Can you work these out from the drawing? Everything is in mm from the part's minimum corner. A direction names the side the tool comes from. Coordinates: 2 decimals unless noted, no trailing zeros. Loops run counter-clockwise (first coordinate to the right, second up) from the corner with the lowest first, then second, coordinate; pieces in that order, holes last. Notation, with made-up numbers: M -23.75,38.25 L 32.25,38.25 A16 cw 32.25,66.25 Z; hole C 67,6 d11. An arc over 180 degrees is marked long. Use CSV: the item, a comma, the result in double quotes. Start each with the question number.
Q1. If we section it at D-D (x = 20.5): Please give me the cut outline in (y, z), and give its area (3 significant figures).
Q2. If we section it at B-B (z = 9.65): Please give me the cut outline in (x, y), and give its area (3 significant figures).
Q3. If we section it at C-C (z = 4.5): Please give me the cut outline in (x, y), and give its area (3 significant figures).
Q4. If we section it at A-A (x = 30.75): Please give me the cut outline in (y, z).
Q5. Which directions (+Z, -Z, +X, -X, +Y, -Y) give clear straight access to the entire face, cutting with the end or side of a thin tool? Please do the marked faces 1 and 2.
Q6. Please list where these lines run through material, in increasing order: probe 1 along Y at (x, z) = (19, 8.25); probe 2 along Y at (x, z) = (30.5, 5.5). Write a range as [from, to].
Q7. For pin 1 Ø1.5 at (x, z) = (23.5, 16.5) entering from -Y, with a flat end and sliding along its axis, tell me the tip position at first contact or that it passes through.
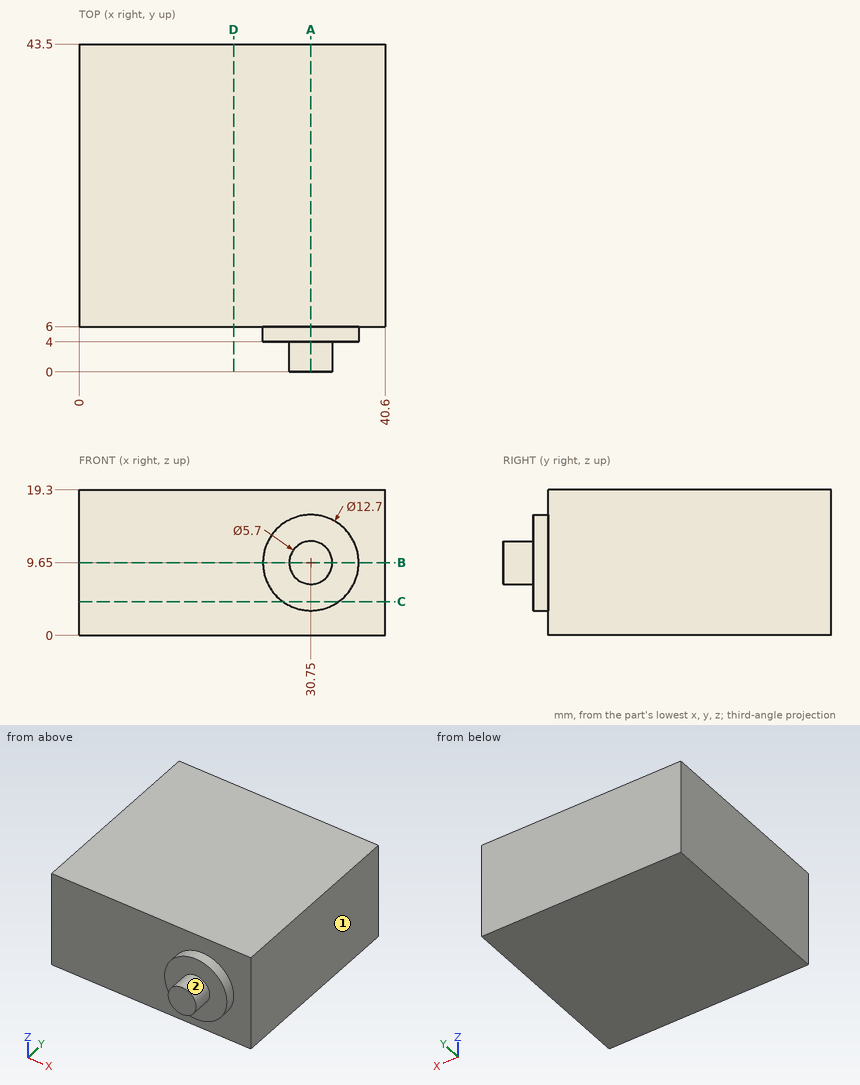
Results below:
1,outline,"M 6,0 L 43.5,0 L 43.5,19.3 L 6,19.3 Z"
1,area,"724 mm^2"
2,outline,"M 0,6 L 24.4,6 L 24.4,4 L 27.9,4 L 27.9,0 L 33.6,0 L 33.6,4 L 37.1,4 L 37.1,6 L 40.6,6 L 40.6,43.5 L 0,43.5 Z"
2,area,"1,570 mm^2"
3,outline,"M 0,6 L 27.04,6 L 27.04,4 L 34.46,4 L 34.46,6 L 40.6,6 L 40.6,43.5 L 0,43.5 Z"
3,area,"1,540 mm^2"
4,outline,"M 0,6.8 L 4,6.8 L 4,3.3 L 6,3.3 L 6,0 L 43.5,0 L 43.5,19.3 L 6,19.3 L 6,16 L 4,16 L 4,12.5 L 0,12.5 Z"
5,face 1,"+Z, -Z, +X, +Y, -Y"
5,face 2,"-Y"
6,probe 1,"[6, 43.5]"
6,probe 2,"[4, 43.5]"
7,pin 1,"y = 6"
